from build123d import *

# Parameters (mm, degrees)
BOSS_EXTRUDE1_DEPTH = 2.54
SKETCH2_W           = 2.54
SKETCH2_H           = 2.54
CUT_EXTRUDE1_DEPTH  = 34.026105205
SKETCH3_W           = 1.27
SKETCH3_H           = 2.032
CUT_EXTRUDE2_DEPTH  = 34.026105205
SKETCH4_W           = 2.54
SKETCH4_H           = 2.54
CUT_EXTRUDE3_DEPTH  = 34.026105205


with BuildPart() as part:
    # Sketch1 → Boss-Extrude1 (new body)
    with BuildSketch(Plane(origin=(0, 0, 0), x_dir=(1, 0, 0), z_dir=(0, 1, 0))):
        Polygon((0, 0), (0, 20.955), (25.4, 20.955), (25.4, 8.255), (12.7, 8.255), (12.7, 0), align=None)
    extrude(amount=BOSS_EXTRUDE1_DEPTH)

    # Sketch2 → Cut-Extrude1 (cut, through all)
    with BuildSketch(Plane(origin=(0, 2.54, 0), x_dir=(1, 0, 0), z_dir=(0, 1, 0))):
        with Locations((3.81, 1.27)):
            Rectangle(SKETCH2_W, SKETCH2_H)
        with Locations((8.89, 1.27)):
            Rectangle(SKETCH2_W, SKETCH2_H)
    extrude(amount=-CUT_EXTRUDE1_DEPTH, mode=Mode.SUBTRACT)

    # Sketch3 → Cut-Extrude2 (cut, through all)
    with BuildSketch(Plane(origin=(0, 2.54, 0), x_dir=(1, 0, 0), z_dir=(0, 1, 0))):
        with Locations((10.16, 16.891)):
            Rectangle(SKETCH3_W, SKETCH3_H)
        with Locations((20.066, 16.891)):
            Rectangle(SKETCH3_W, SKETCH3_H)
    extrude(amount=-CUT_EXTRUDE2_DEPTH, mode=Mode.SUBTRACT)

    # Sketch4 → Cut-Extrude3 (cut, through all)
    with BuildSketch(Plane(origin=(0, 2.54, 0), x_dir=(1, 0, 0), z_dir=(0, 1, 0))):
        with Locations((1.27, 6.35)):
            Rectangle(SKETCH4_W, SKETCH4_H)
        with Locations((11.43, 6.35)):
            Rectangle(SKETCH4_W, SKETCH4_H)
    extrude(amount=-CUT_EXTRUDE3_DEPTH, mode=Mode.SUBTRACT)


solid = part.part
Verification items for the finished model (mm, model axes). A direction names the side the tool comes from. Coordinates: 2 decimals unless noted, no trailing zeros. Order: outer loops, then holes, each group sorted by start corner. A loop starts at its lowest first (then second) coordinate and runs counter-clockwise, first axis right, second up. Notation, with made-up numbers: (60.25, 37) -> (66.25, 37) arc R12 ccw to (66.25, 41) -> close; hole circle Ø10 at (-16, 74). An arc over 180 degrees is marked (long way). Put each result on its own line as item: value. Start each with the question number.
1. Cross-section at C-C, the plane x = 20. Record the boundary of the cut face in (y, z) (3 decimals), then the cut area to 3 significant figures.
2. Access from +Z, -Z, +X, -X, +Y, -Y to the whole of each face (thin tool, end or side, straight path). Record for faces 4 (the flat face through (7.62, 1, -1)), 5 (the flat face through (11, 1, -7.62)), 6 (the flat face through (2.54, 1, -6)).
3. Cross-section at A-A, the plane y = 2.2. Count the separate pieces of the cut face and the enclosed holes in it, then the cut area to 3 significant figures.
4. Go/stop test with flat-tipped pins: pin 1 Ø0.8 at (y, z) = (1.5, -1.5) entering from +X; pin 2 Ø1.3 at (x, y) = (3.5, 1) entering from +Z; pin 3 Ø0.8 at (y, z) = (1, -6) entering from +X. Record where each tip stops, or that it passes through.
5. Cross-section at B-B, the plane z = -1.5. Record the boundary of the cut face in (x, y), then the cut area to 3 significant figures.
6. Material ranges on L1, parallel to X at y = 2.2, z = -16 (3 decimals); L2, parallel to X at y = 0.1, z = -2; L3, parallel to Z at x = 10.5, y = 0.5 (3 decimals), recorded low to high. Write a range as [from, to].
7. Mould release check, pull along X, two halves, no side actions. Record for faces 1 (the flat face through (25.4, 1, -15)), 2 (the flat face through (6, 1, 0)), 3 (the flat face through (20.701, 1, -17)): released by +X, released by -X, zero draft, split by the parting line, or undercut.
8. Cross-section at D-D, the plane z = -6.5. Record the boundary of the cut face in (x, y), then the cut area to 3 significant figures.
Computed:
1. outline: (0, -20.955) -> (2.54, -20.955) -> (2.54, -17.907) -> (0, -17.907) -> close; (0, -15.875) -> (2.54, -15.875) -> (2.54, -8.255) -> (0, -8.255) -> close
1. area: 27.1 mm2
2. face 4: +Z, +Y, -Y
2. face 5: +X, +Y, -Y
2. face 6: -X, +Y, -Y
3. separate pieces: 1
3. enclosed holes: 2
3. area: 396 mm2
4. pin 1: x = 12.7
4. pin 2: z = -2.54
4. pin 3: x = 10.16
5. outline: (0, 0) -> (2.54, 0) -> (2.54, 2.54) -> (0, 2.54) -> close; (5.08, 0) -> (7.62, 0) -> (7.62, 2.54) -> (5.08, 2.54) -> close; (10.16, 0) -> (12.7, 0) -> (12.7, 2.54) -> (10.16, 2.54) -> close
5. area: 19.4 mm2
6. L1: [0, 9.525], [10.795, 19.431], [20.701, 25.4]
6. L2: [0, 2.54], [5.08, 7.62], [10.16, 12.7]
6. L3: [-20.955, -17.907], [-15.875, -7.62], [-5.08, 0]
7. face 1: released by +X
7. face 2: zero draft
7. face 3: undercut
8. outline: (2.54, 0) -> (10.16, 0) -> (10.16, 2.54) -> (2.54, 2.54) -> close
8. area: 19.4 mm2
